Autodesk Inventor part; units mm, degrees
ref_plane "YZ Plane" through (0, 0, 0) normal (1, 0, 0) x (0, 1, 0)
ref_plane "XZ Plane" through (0, 0, 0) normal (0, 1, 0) x (-1, 0, 0)
ref_plane "XY Plane" through (0, 0, 0) normal (0, 0, 1) x (1, 0, 0)
sketch "Sketch1" plane through (0, 0, 0) normal (0, 0, 1) x (1, 0, 0)
  line L0 (-12.4598, 60) -> (12.4598, 60)
  line L1 (-22.4598, -14.4802) -> (-22.4598, 50)
  arc A0 (-12.4598, 60) -> (-22.4598, 50) centre (-12.4598, 50) ccw
  arc A1 (22.4598, 50) -> (12.4598, 60) centre (12.4598, 50) ccw
  line L2 (27.4598, -2.8868) -> (70.0912, -27.5)
  line L3 (22.4598, 0) -> (71.6863, 0) construction
  line L4 (73.7514, -41.1603) -> (63.7514, -58.4808)
  line L5 (50.0912, -62.141) -> (-17.4598, -23.1405)
  line L6 (22.4598, 50) -> (22.4598, 5.7735)
  arc A2 (-22.4598, -14.4802) -> (-17.4598, -23.1405) centre (-12.4598, -14.4802) ccw
  arc A3 (22.4598, 5.7735) -> (27.4598, -2.8868) centre (32.4598, 5.7735) ccw
  arc A4 (73.7514, -41.1603) -> (70.0912, -27.5) centre (65.0912, -36.1603) ccw
  arc A5 (50.0912, -62.141) -> (63.7514, -58.4808) centre (55.0912, -53.4808) ccw
  point P0 (0, 0)
  point P1 (0, 60)
  point P2 (78.7514, -32.5)
  point P3 (58.7514, -67.141)
  dimension "d0" = 10
  dimension "d11" = 65
  dimension "d12" = 30
  dimension "d13" = 40
  dimension "d14" = 10
extrude "Extrusion1" add sketch "Sketch1" along normal blind 5
sketch "Sketch2" plane through (0, 0, 5) normal (0, 0, 1) x (1, 0, 0)
  circle A0 centre (0, 50) radius 5
  line L0 (-22.4598, 50) -> (-22.4598, -14.4802) construction
  line L1 (-22.4598, 17.7599) -> (22.4598, 27.8868) construction
  line L2 (22.4598, 5.7735) -> (22.4598, 50) construction
  line L3 (12.4598, 60) -> (-12.4598, 60)
  circle A1 centre (0, -10) radius 5
  line L4 (63.7514, -58.4808) -> (73.7514, -41.1603)
  ellipse E0 centre (42.7707, -34.8205) end of major axis (63.7179, -46.9144) minor radius 13.5207
  line L5 (70.0912, -27.5) -> (27.4598, -2.8868)
  point P0 (0, 0)
  point P1 (0, 22.8233)
  dimension "d5" = 10
  dimension "d7" = 10
  dimension "d15" = 10
  dimension "d16" = 10
  dimension "d19" = 30
  dimension "d20" = 20
extrude "Extrusion2" cut sketch "Sketch2" against normal up to surface (5 mm away)
properties part number "base"
Could you check a few things on this model? Use its own coordinates, in mm. A direction names the side the tool comes from. Round coordinates to 2 decimals unless told otherwise and drop trailing zeros. Loops run counter-clockwise (first coordinate to the right, second up) from the corner with the lowest first, then second, coordinate; pieces in that order, holes last. Notation, with made-up numbers: (-33.75, 37.5) - (-12.75, 37.5) arc R10 ccw to (-12.75, 43.5) - close; hole circle Ø8 at (-16.75, 15). An arc over 180 degrees is marked (long way). Answer as CSV lines item,"result".
1. I want a section at B-B on x = 0. List the corners of the cut face in (y, z) for me.
Filled in:
outline,"(-33.22, 0) - (-15, 0) - (-15, 5) - (-33.22, 5) - close; (-5, 0) - (45, 0) - (45, 5) - (-5, 5) - close; (55, 0) - (60, 0) - (60, 5) - (55, 5) - close"
2. Please list where these lines run through material, in increasing order: line 1 along Y through (x, z) = (0, 1.3); line 2 along Y through (x, z) = (3.5, 1.05); line 3 along X through (y, z) = (38, 4). Write a range as [from, to].
Filled in:
line 1,"y = [-33.22, -15], [-5, 45], [55, 60]"
line 2,"y = [-35.24, -13.57], [-6.43, 46.43], [53.57, 60]"
line 3,"x = [-22.46, 22.46]"
3. I want a section at C-C on y = -10. List the corners of the cut face in (x, z) for me.
Filled in:
outline,"(-22.46, 0) - (-5, 0) - (-5, 5) - (-22.46, 5) - close; (5, 0) - (39.78, 0) - (39.78, 5) - (5, 5) - close"
4. I want a section at D-D on z = 3.8. Count the separate pieces of the cut face and the enclosed holes in it, then the cut area to 3 significant figures.
Filled in:
separate pieces,"1"
enclosed holes,"3"
area,"5,060 mm^2"
5. I want a section at A-A on y = 52.5. List the corners of the cut face in (x, z) for me.
Filled in:
outline,"(-22.14, 0) - (-4.33, 0) - (-4.33, 5) - (-22.14, 5) - close; (4.33, 0) - (22.14, 0) - (22.14, 5) - (4.33, 5) - close"
6. We'd pull the mould along X, two halves only. Please class faces 3 (the face through (-0.651, -5.043, 2.535)), 4 (the face through (-21.083, -19.544, 2.465)), 5 (the face through (15, -1, 0)): +X half, -X half, draft (parallel to the pull), parting line (faces both ways), or undercut.
Filled in:
face 3,"undercut"
face 4,"-X half"
face 5,"draft"
7. For pin 1 Ø2 at (x, z) = (56.5, 4.5) entering from +Y; pin 2 Ø2 at (x, z) = (24.5, 3.5) entering from +Y; pin 3 Ø16 at (x, y) = (0, 50) entering from +Z; pin 4 Ø1.5 at (y, z) = (-6, 4.5) entering from +X, each with a flat end and sliding along its axis, tell me the tip position at first contact or that it passes through.
Filled in:
pin 1,"stops at y = -19.08"
pin 2,"stops at y = 1.33"
pin 3,"stops at z = 5"
pin 4,"stops at x = 34.15"
8. On a 3-axis mill with a long thin cutter (end or side, diameter ignored), from which of +Z, -Z, +X, -X, +Y, -Y can I reach the whole of each face in a straight line? I mean faces 1 (the face through (22.46, 28, 2)), 2 (the face through (57.79, -63.11, 2.46)). Say none if no direction works.
Filled in:
face 1,"+Z, -Z, +X, +Y"
face 2,"+Z, -Z, -Y"
